```python
from build123d import *

# Parameters (mm, degrees)
BOSS_EXTRUDE1_DEPTH = 15


with BuildPart() as part:
    # Sketch1 → Boss-Extrude1 (new body)
    with BuildSketch(Plane(origin=(0, 0, 0), x_dir=(0, 0, -1), z_dir=(1, 0, 0))):
        Polygon((30.824095604, 67.060925147), (30.824095604, 21.060925147), (40.824095604, 21.060925147), (40.824095604, 77.060925147), (-4.175904396, 77.060925147), (-4.175904396, -52.939074853), (5.824095604, -52.939074853), (5.824095604, 67.060925147), align=None)
        Polygon((-4.175904396, -52.939074853), (-4.175904396, -42.939074853), (-24.175904396, -42.939074853), (-24.175904396, -12.939074853), (-34.175904396, -12.939074853), (-34.175904396, -52.939074853), align=None)
    extrude(amount=BOSS_EXTRUDE1_DEPTH)


solid = part.part
```
Part model, mm, in its own coordinate system. A direction names the side the tool comes from. Give positions to 0.01 mm unless a question says otherwise; leave off trailing zeros. Order: outer loops, then holes, each group sorted by start corner. A loop starts at its lowest first (then second) coordinate and runs counter-clockwise, first axis right, second up. Notation, with made-up numbers: M -23,-26 L -13,-26 A25 ccw -13,3 Z; hole C 13,48.25 d4. An arc over 180 degrees is marked long. Use a Markdown table: item, result. Add a question column.
(1) Saw through at A-A, the plane y = -31.5. Give the cut face in (x, z), and give its area (3 significant figures).
(2) Drop flat-ended pins along their axis: P1, Ø7.5, axis at x = 9, y = -31, coming from the -Z side; P2, Ø3, axis at x = 4, z = -35.5, coming from the -Y side; P3, Ø2, axis at x = 7, y = 58, coming from the +Z side. Give the stop position or say it passes through.
(3) Mould opens along Z. For faces 1 (the face through (7, 18, 4.176)), 2 (the face through (7, 49, -40.824)), 3 (the face through (7, 21.061, -36)) say: +Z half, -Z half, draft (parallel to the pull), parting line (faces both ways), or undercut.
(4) Saw through at D-D, the plane y = 5. Give the cut face in (x, z).
(5) Probe line 1 along Z through (x, y) = (8.75, 44); line 2 along Z through (x, y) = (12.75, -30.5); line 3 along Z through (x, y) = (5, 17). List the from-to ranges inside material, lowest first. Write a range as [from, to].
(6) Saw through at B-B, the plane x = 7. Give the cut face in (y, z).
(7) 3-axis set-ups, long thin cutter, end or side, ignore diameter. For faces 4 (the face through (7, -42.939, 14)), 5 (the face through (15, 17, -3)), 6 (the face through (7, -52.939, 14)), 7 (the face through (7, 6, -5.824)), 8 (the face through (7, -12.939, 29)): which of +Z, -Z, +X, -X, +Y, -Y reach the whole face in a straight line?
(8) Saw through at C-C, the plane z = 10. Give the cut face in (x, y).
Answer key:
| question | item | result |
|---|---|---|
| 1 | outline | M 0,-5.82 L 15,-5.82 L 15,4.18 L 0,4.18 Z; M 0,24.18 L 15,24.18 L 15,34.18 L 0,34.18 Z |
| 1 | area | 300 mm^2 |
| 2 | P1 | z = -5.82 |
| 2 | P2 | y = 21.06 |
| 2 | P3 | z = 4.18 |
| 3 | face 1 | undercut |
| 3 | face 2 | -Z half |
| 3 | face 3 | draft |
| 4 | outline | M 0,-5.82 L 15,-5.82 L 15,4.18 L 0,4.18 Z |
| 5 | line 1 | [-40.82, -30.82], [-5.82, 4.18] |
| 5 | line 2 | [-5.82, 4.18], [24.18, 34.18] |
| 5 | line 3 | [-5.82, 4.18] |
| 6 | outline | M -52.94,-5.82 L 67.06,-5.82 L 67.06,-30.82 L 21.06,-30.82 L 21.06,-40.82 L 77.06,-40.82 L 77.06,4.18 L -42.94,4.18 L -42.94,24.18 L -12.94,24.18 L -12.94,34.18 L -52.94,34.18 Z |
| 7 | face 4 | +X, -X, +Y |
| 7 | face 5 | +Z, -Z, +X, +Y, -Y |
| 7 | face 6 | +Z, -Z, +X, -X, -Y |
| 7 | face 7 | +X, -X, -Y |
| 7 | face 8 | +Z, +X, -X, +Y |
| 8 | outline | M 0,-52.94 L 15,-52.94 L 15,-42.94 L 0,-42.94 Z |
